Read the model definition and answer for the solid it produces. Units are mm, in the model's axes. Round coordinates to 2 decimals unless told otherwise and drop trailing zeros. Write each loop counter-clockwise with the first axis right and the second up, starting at its lowest first coordinate (ties: lowest second). Pieces come first, ordered by that corner, then holes. Notation, with made-up numbers: (19, -23) - (23, -23) arc R12 cw to (23, -15) - close; hole circle Ø3 at (32.25, 28). An arc over 180 degrees is marked (long way). One line per item, written item: value. Start each with the question number.
(1) A cutting plane is placed at A-A, the plane x = -95.25. Determine the outline of the cut face in (y, z).
(2) The mould has two halves that part along Y. Classify faces 1 (the face through (13.904, 58.076, 9.392)), 2 (the face through (-2, -101.6, 9)), 3 (the face through (107.95, -1, 9)): +Y half, -Y half, draft (parallel to the pull), parting line (faces both ways), or undercut.
(3) Find the intervals of material crossed by L1, parallel to Y at x = 12.7, z = 11.5; L2, parallel to X at y = 62, z = 16.5; L3, parallel to X at y = 66, z = 7, in increasing order.
(4) A cutting plane is placed at B-B, the plane x = 12.7. Determine the outline of the cut face in (y, z).
from build123d import *

# Parameters (mm, degrees)
F0_W     = 215.9
F0_H     = 203.2
F1_DEPTH = 19.05
F3_D     = 7.9375
F4_D     = 11.1125


# Not quite as in the source:
# - a length typed as a fraction of an inch, garbled in the dataset ("3 / 203.2 mm" for 3/8 in), is restored


with BuildPart() as f1:
    # F0 (on Top) → F1 (new body)
    with BuildSketch(Plane.XY):
        Rectangle(F0_W, F0_H)
    extrude(amount=F1_DEPTH)

    # F3 (through all)
    with Locations(Plane.XY.offset(19.05)):
        with Locations((-95.25, 60.452), (-55.626, 60.452), (-95.25, -60.452), (-55.626, -60.452)):
            Hole(F3_D / 2)

    # F4 (through all)
    with Locations(Plane.XY.offset(19.05)):
        with Locations((12.7, 63.5), (88.9, 63.5), (12.7, -63.5), (88.9, -63.5)):
            Hole(F4_D / 2)


solid = f1.part
Here are the results:
1. outline: (-101.6, 0) - (-64.42, 0) - (-64.42, 19.05) - (-101.6, 19.05) - close; (-56.48, 0) - (56.48, 0) - (56.48, 19.05) - (-56.48, 19.05) - close; (64.42, 0) - (101.6, 0) - (101.6, 19.05) - (64.42, 19.05) - close
2. face 1: undercut
2. face 2: -Y half
2. face 3: draft
3. L1: -101.6 to -69.06, -57.94 to 57.94, 69.06 to 101.6
3. L2: -107.95 to -98.9, -91.6 to -59.28, -51.97 to 7.35, 18.05 to 83.55, 94.25 to 107.95
3. L3: -107.95 to 7.74, 17.66 to 83.94, 93.86 to 107.95
4. outline: (-101.6, 0) - (-69.06, 0) - (-69.06, 19.05) - (-101.6, 19.05) - close; (-57.94, 0) - (57.94, 0) - (57.94, 19.05) - (-57.94, 19.05) - close; (69.06, 0) - (101.6, 0) - (101.6, 19.05) - (69.06, 19.05) - close
